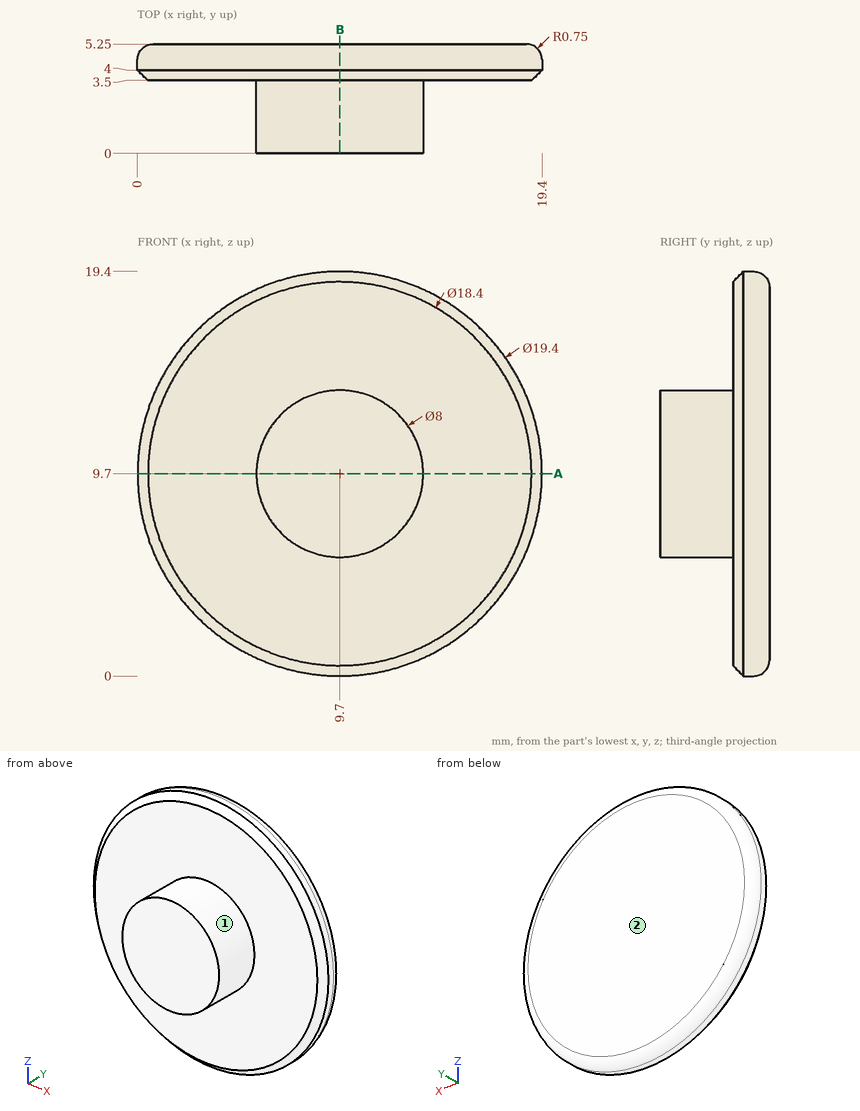
Could you check a few things on this drawing? It's one solid part, dimensions in mm from its lowest x, y, z. A direction names the side the tool comes from. Give positions to 0.01 mm unless a question says otherwise; leave off trailing zeros. Order: outer loops, then holes, each group sorted by start corner. A loop starts at its lowest first (then second) coordinate and runs counter-clockwise, first axis right, second up. Notation, with made-up numbers: M 48.5,9.25 L 70.5,9.25 A16 ccw 70.5,21.25 Z; hole C -25.5,80.25 d9. An arc over 180 degrees is marked long. Use one line per item in the form item = value.
Item 1: If we section it at A-A, the plane z = 9.7: Write out the boundary of the cut face in (x, y), and give its area (3 significant figures).
Values follow:
outline = M 0,4 L 0.5,3.5 L 5.7,3.5 L 5.7,0 L 13.7,0 L 13.7,3.5 L 18.9,3.5 L 19.4,4 L 19.4,4.5 A0.75 ccw 18.65,5.25 L 0.75,5.25 A0.75 ccw 0,4.5 Z
area = 61.5 mm^2
Item 2: Will these pins go through, and if not, where does the flat tip stop? pin 1 Ø1 at (y, z) = (1.5, 7) entering from +X; pin 2 Ø3 at (x, y) = (3, 3.5) entering from -Z.
Values follow:
pin_1 = 13.04
pin_2 = 1.57
Item 3: If I drill on line 1 along Y through (x, z) = (5, 12.25); line 2 along X through (y, z) = (0.3, 11.25); line 3 along X through (y, z) = (0.35, 11.5), over which ranges is the centre line in solid material (lowest first)? Write a range as [from, to].
Values follow:
line_1 = [3.5, 5.25]
line_2 = [6.01, 13.39]
line_3 = [6.13, 13.27]
Item 4: For the marked faces 1 and 2, which set-ups out of +Z, -Z, +X, -X, +Y, -Y let a thin tool reach every point of the face, with its end or its side?
Values follow:
face_1 = -Y
face_2 = +Z, -Z, +X, -X, +Y
Item 5: If we section it at B-B, the plane x = 9.7: Write out the boundary of the cut face in (y, z), and give its area (3 significant figures).
Values follow:
outline = M 0,5.7 L 3.5,5.7 L 3.5,0.5 L 4,0 L 4.5,0 A0.75 ccw 5.25,0.75 L 5.25,18.65 A0.75 ccw 4.5,19.4 L 4,19.4 L 3.5,18.9 L 3.5,13.7 L 0,13.7 Z
area = 61.5 mm^2
